Can you work these out from the drawing? Everything is in mm from the part's minimum corner. Coordinates: 2 decimals unless noted, no trailing zeros. Loops run counter-clockwise (first coordinate to the right, second up) from the corner with the lowest first, then second, coordinate; pieces in that order, holes last. Notation, with made-up numbers: (21, 24) - (51, 24) arc R11 cw to (51, 38) - close; hole circle Ø7 at (35, 1.5). An arc over 180 degrees is marked (long way). One line per question, with ' | ' between items. Start each with the question number.
1. I want a section at D-D, the plane y = 102. Write out the boundary of the cut face in (x, z).
2. I want a section at B-B, the plane x = 102. Write out the boundary of the cut face in (y, z).
3. I want a section at C-C, the plane x = 262. Write out the boundary of the cut face in (y, z).
4. I'm going to push flat-ended pins straight in: P1, Ø1.1, axis at y = 58, z = 1.5, coming from the +X side; P2, Ø1.8, axis at y = 2.5, z = 1, coming from the +X side; P3, Ø1.8, axis at x = 278, z = 2, coming from the -Y side; P4, Ø12, axis at x = 240, y = 79.5, coming from the +Z side. Where does each tip first touch, or does it pass through?
5. Please list where these lines run through material, in increasing order: L1, parallel to Y at x = 236, z = 1; L2, parallel to Y at x = 134.5, z = 1.35; L3, parallel to X at y = 59, z = 3.25. Write a range as [from, to].
6. I want a section at A-A, the plane y = 71.5. Write out the boundary of the cut face in (x, z), then the cut area to 3 significant figures.
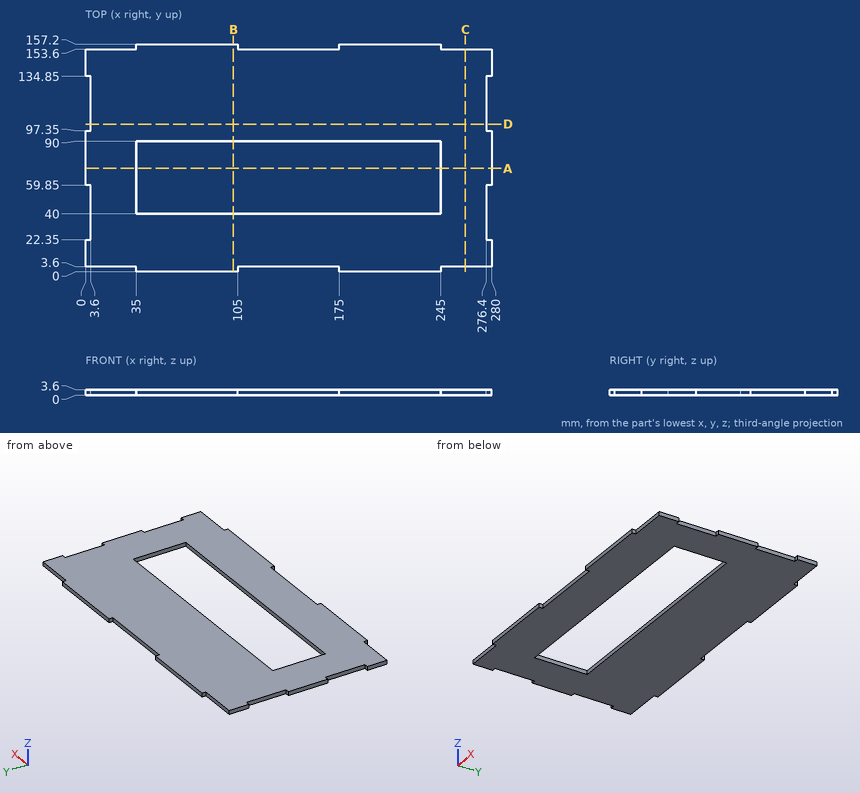
Results are:
1) outline: (3.6, 0) - (276.4, 0) - (276.4, 3.6) - (3.6, 3.6) - close
2) outline: (0, 0) - (40, 0) - (40, 3.6) - (0, 3.6) - close; (90, 0) - (157.2, 0) - (157.2, 3.6) - (90, 3.6) - close
3) outline: (3.6, 0) - (153.6, 0) - (153.6, 3.6) - (3.6, 3.6) - close
4) P1: stops at x = 276.4 | P2: stops at x = 245 | P3: stops at y = 3.6 | P4: stops at z = 3.6
5) L1: y = [0, 40], [90, 157.2] | L2: y = [3.6, 40], [90, 153.6] | L3: x = [3.6, 35], [245, 276.4]
6) outline: (0, 0) - (35, 0) - (35, 3.6) - (0, 3.6) - close; (245, 0) - (280, 0) - (280, 3.6) - (245, 3.6) - close | area: 252 mm2
